Input: dimensioned drawing with shaded views. Units: mm. Origin: part minimum x, y, z. Give positions to 0.01 mm unless a question says otherwise; leave off trailing zeros. Write each loop counter-clockwise with the first axis right and the second up, starting at its lowest first coordinate (ties: lowest second). Pieces come first, ordered by that corner, then holes.
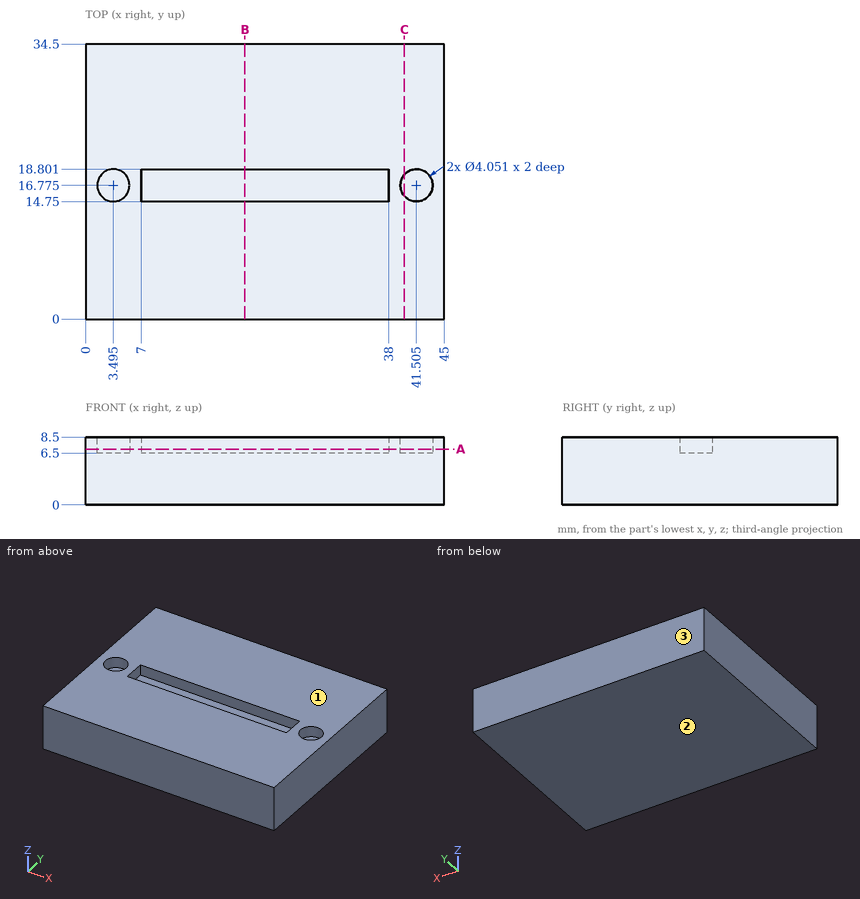
Item 1: Pin query (flat end, axial travel): pin 1 (2 mm diameter, centred on x = 3, y = 16.5, fed in from +Z). Return the tip coordinate at first contact, or that it passes through.
Item 2: Section C-C (x = 40). Return loops of the section in (y, z).
Item 3: Section A-A (z = 7). Give the number of separate pieces and of enclosed holes in the cut face, and give its area (3 significant figures).
Item 4: Mould query, pull axis Z, two halves, no side actions, for the marked faces 1, 2 and 3. Classes: +Z half, -Z half, draft (parallel to the pull), parting line (faces both ways), or undercut.
Item 5: Ray query, line 1 (Y direction, x = 13.5, z = 6.75). Return the intervals inside material, ascending.
Item 6: Section B-B (x = 20). Return loops of the section in (y, z).
Solved:
1. pin 1: stops at z = 6.5
2. outline: (0, 0) - (34.5, 0) - (34.5, 8.5) - (18.13, 8.5) - (18.13, 6.5) - (15.42, 6.5) - (15.42, 8.5) - (0, 8.5) - close
3. separate pieces: 1
3. enclosed holes: 3
3. area: 1,400 mm2
4. face 1: +Z half
4. face 2: -Z half
4. face 3: draft
5. line 1: y = 0 to 14.75, 18.8 to 34.5
6. outline: (0, 0) - (34.5, 0) - (34.5, 8.5) - (18.8, 8.5) - (18.8, 6.5) - (14.75, 6.5) - (14.75, 8.5) - (0, 8.5) - close
